Geometry: final body of the model. Coordinates: model frame, mm. Face numbers are marked on the shaded views. A direction names the side the tool comes from. Round coordinates to 2 decimals unless told otherwise and drop trailing zeros. Loops run counter-clockwise (first coordinate to the right, second up) from the corner with the lowest first, then second, coordinate; pieces in that order, holes last. Notation, with made-up numbers: (63.5, -15) - (115.5, -15) arc R16 cw to (115.5, -8) - close; hole circle Ø3 at (59.25, 33). An arc over 180 degrees is marked (long way). Answer as CSV lines item,"result".
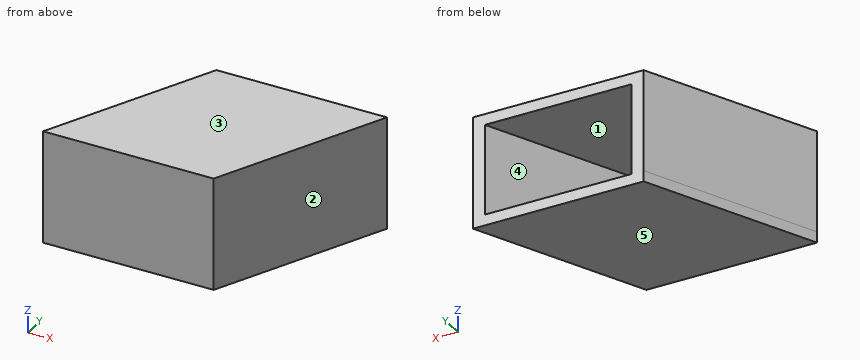
from build123d import *

# Parameters (mm, degrees)
F1_DEPTH = 20.8
F3_DEPTH = 2.5
F4_START = -23.3
F4_DEPTH = 2.5


with BuildPart() as f1:
    # F0 (on Top) → F1 (new body)
    with BuildSketch(Plane.XY):
        Polygon((33.984039904, 0), (0, 0), (16.3207680354, 35), (13.562323238, 35), (-4.62367543, -4), (34.8772540688, -4), (53.0632527369, 35), (50.3048079395, 35), align=None)
    extrude(amount=F1_DEPTH)

    # F2 (on face) → F3 (join)
    with BuildSketch(Plane.XY.offset(20.8)):
        Polygon((50.3048079395, 35), (16.3207680354, 35), (0, 0), (33.984039904, 0), align=None)
        Polygon((16.3207680354, 35), (13.562323238, 35), (-4.62367543, -4), (34.8772540688, -4), (53.0632527369, 35), (50.3048079395, 35), (33.984039904, 0), (0, 0), align=None)
    extrude(amount=F3_DEPTH)

    # F3_face (on face) → F4 (join)
    with BuildSketch(Plane(origin=(24.2197886534, 15.5, 23.3), x_dir=(1, 0, 0), z_dir=(0, 0, 1)).offset(F4_START)):
        Polygon((-10.6574654154, 19.5), (-28.8434640835, -19.5), (10.6574654154, -19.5), (28.8434640835, 19.5), align=None)
    extrude(amount=-F4_DEPTH)


solid = f1.part
(1) Section A-A (z = 3.75). Output: boundary loops of the cut face in (x, y), and give its area (3 significant figures).
Findings below:
outline,"(-4.62, -4) - (34.88, -4) - (53.06, 35) - (50.3, 35) - (33.98, 0) - (0, 0) - (16.32, 35) - (13.56, 35) - close"
area,"351 mm2"
(2) Material intervals for line 1 along Z through (x, y) = (28.5, 3.5); line 2 along Y through (x, z) = (29, 19.25); line 3 along X through (y, z) = (16, 3), sorted ascending.
Findings below:
line 1,"-2.5 to 0, 20.8 to 23.3"
line 2,"-4 to 0"
line 3,"4.7 to 7.46, 41.44 to 44.2"
(3) Section B-B (x = 18). Output: boundary loops of the cut face in (y, z), and give its area (3 significant figures).
Findings below:
outline,"(-4, -2.5) - (35, -2.5) - (35, 0) - (0, 0) - (0, 20.8) - (35, 20.8) - (35, 23.3) - (-4, 23.3) - close"
area,"278 mm2"
(4) Access query for the marked faces 4 and 5. Directions: +Z, -Z, +X, -X, +Y, -Y. A direction counts if a zero-diameter tool reaches every point of the face in a straight line with its end or side. Return the directions, or none.
Findings below:
face 4,"+Y"
face 5,"-Z, +X, -X, +Y, -Y"
(5) Section D-D (x = 9.5). Output: boundary loops of the cut face in (y, z).
Findings below:
outline,"(-4, -2.5) - (26.29, -2.5) - (26.29, 23.3) - (-4, 23.3) - close; hole (0, 0) - (20.37, 0) - (20.37, 20.8) - (0, 20.8) - close"
(6) Draft query along X for the marked faces 1, 2 and 3. Return one class per face: pulls with the +X half, pulls with the -X half, needs draft (parallel to the pull), parting line crosses it, or undercut.
Findings below:
face 1,"undercut"
face 2,"pulls with the +X half"
face 3,"needs draft"
(7) Section C-C (y = 6). Output: boundary loops of the cut face in (x, z), and give its area (3 significant figures).
Findings below:
outline,"(0.04, -2.5) - (39.54, -2.5) - (39.54, 23.3) - (0.04, 23.3) - close; hole (2.8, 0) - (36.78, 0) - (36.78, 20.8) - (2.8, 20.8) - close"
area,"312 mm2"
(8) Pin query (flat end, axial travel): P1, Ø4, axis at y = 6.5, z = 16, coming from the -X side; P2, Ø12, axis at y = 23, z = 16.5, coming from the +X side; P3, Ø2, axis at y = 21, z = 5, coming from the +X side. Return the tip coordinate at first contact, or that it passes through.
Findings below:
P1,"x = -0.66"
P2,"x = 50.27"
P3,"x = 47"
